The model under review builds one solid part; all positions refer to its coordinate system, in mm. Round coordinates to 2 decimals unless told otherwise and drop trailing zeros. Order: outer loops, then holes, each group sorted by start corner. A loop starts at its lowest first (then second) coordinate and runs counter-clockwise, first axis right, second up.
```python
from build123d import *

# Parameters (mm, degrees)
F0_R     = 2.5
F1_DEPTH = 2
F2_SIZE  = 0.5
F3_R     = 0.5


with BuildPart() as f1:
    # F0 (on Front) → F1 (new body)
    with BuildSketch(Plane.XZ):
        with BuildLine():
            Line((-9.862112, 18.225786), (-23.862112, 18.225786))
            ThreePointArc((-23.862112, 18.225786), (-29.362112, 12.725786), (-23.862112, 7.225786))
            Line((-23.862112, 7.225786), (-9.862112, 7.225786))
            ThreePointArc((-9.862112, 7.225786), (-4.362112, 12.725786), (-9.862112, 18.225786))
        make_face()
        with Locations((-23.862112, 12.725786)):
            Circle(F0_R, mode=Mode.SUBTRACT)
        with Locations((-9.862112, 12.725786)):
            Circle(F0_R, mode=Mode.SUBTRACT)
    extrude(amount=F1_DEPTH)

    # F2
    f2_edges = [f1.edges().sort_by_distance(p)[0] for p in [
        (-26.362112, -2, 12.725786),
        (-26.362112, 0, 12.725786),
        (-12.362112, -2, 12.725786),
        (-12.362112, 0, 12.725786),
    ]]
    chamfer(f2_edges, length=F2_SIZE)

    # F3
    f3_edges = [f1.edges().sort_by_distance(p)[0] for p in [
        (-16.862112, -2, 7.225786),
        (-29.362112, 0, 12.725786),
    ]]
    fillet(f3_edges, radius=F3_R)


solid = f1.part
```
(1) Consider section A-A (z = 15). State how many separate pieces and enclosed holes the cut face has, and give its area (3 significant figures).
Data:
separate pieces: 3
enclosed holes: 0
area: 37.5 mm2
(2) Consider section B-B (y = -1.15). Write out the cut boundary in (x, z).
Data:
outline: (-23.86, 7.23) - (-9.86, 7.23) arc R5.5 ccw to (-9.86, 18.23) - (-23.86, 18.23) arc R5.5 ccw to start; hole circle Ø5 at (-23.86, 12.73); hole circle Ø5 at (-9.86, 12.73)
(3) Insertion check: pin 1 (6.5 mm diameter, centred on x = -23.86, z = 12.73, fed in from -Y); pin 2 (1 mm diameter, centred on x = -25.5, y = -0.5, fed in from +Z). Each pin has a flat end and moves straight along its axis. Give the tip position at first contact, or say it passes through.
Data:
pin 1: stops at y = -2
pin 2: stops at z = 18.11
(4) Draft analysis for pull direction Z (two halves, no side actions). For faces 1 (the flat face through (-17, -1, 18.226)), 2 (the flat face through (-17, -2, 13)), 3 (the cylindrical face through (-10.188, -0.993, 15.205)), state which applies: pulls with the +Z half, pulls with the -Z half, needs draft (parallel to the pull), parting line crosses it, or undercut.
Data:
face 1: pulls with the +Z half
face 2: needs draft
face 3: undercut
(5) To check wall thickness, follow probe 1 along X at (y, z) = (-0.6, 12.25); probe 2 along X at (y, z) = (-0.6, 14); probe 3 along Z at (x, y) = (-24.25, -0.8). State the ranges of each line that lie inside material, in increasing order.
Data:
probe 1: x = -29.34 to -26.32, -21.41 to -12.32, -7.41 to -4.38
probe 2: x = -29.21 to -26.01, -21.71 to -12.01, -7.71 to -4.51
probe 3: z = 7.24 to 10.26, 15.2 to 18.21
